Study the drawing (mm; zero at the part's minimum x, y, z) and answer. A direction names the side the tool comes from. Coordinates: 2 decimals unless noted, no trailing zeros. Order: outer loops, then holes, each group sorted by start corner. A loop starts at its lowest first (then second) coordinate and runs counter-clockwise, first axis right, second up. Notation, with made-up numbers: M -12.5,-35 L 22.5,-35 A27 cw 22.5,-8 Z; hole C 88,20 d9. An arc over 180 degrees is marked long. Use a Markdown table: item, result. Add a question column.
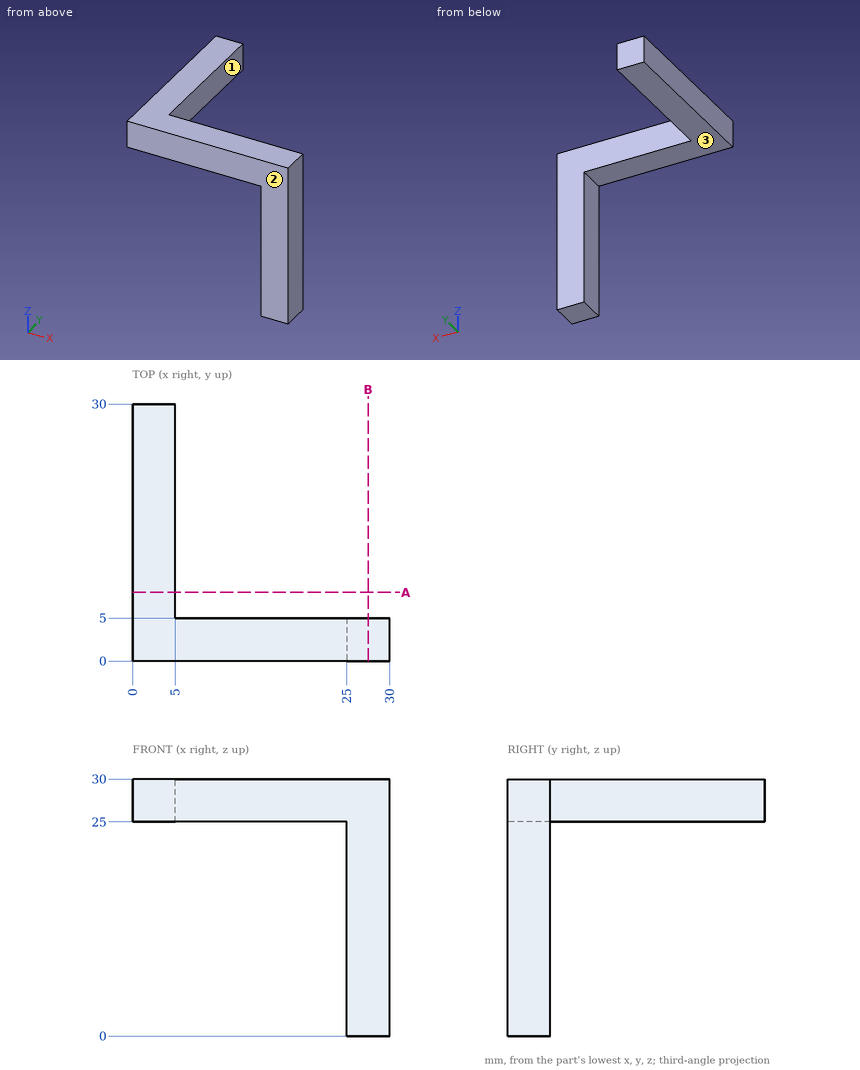
(1) A cutting plane is placed at A-A on y = 8. Write down the section's boundary in (x, z).
(2) Given P1, Ø2, axis at x = 20, y = 6.5, coming from the -Z side; P2, Ø5.5, axis at y = 2.5, z = 6.5, coming from the -X side; P3, Ø3, axis at x = 25.5, z = 14, coming from the +Y side; P4, Ø5.5, axis at y = 15.5, z = 28, coming from the +X side, each flat-ended and moving along its own axis, determine where each tip first touches the part or whether it passes through.
(3) Which of the six approach directions +Z, -Z, +X, -X, +Y, -Y give full straight-line access (tool end or side, diameter ignored) to the marked faces 1, 2 and 3?
(4) A cutting plane is placed at B-B on x = 27.5. Write down the section's boundary in (y, z).
(5) Straight lines are drawn through the part: line 1 (Y direction, x = 20.25, z = 25.5); line 2 (Z direction, x = 1.75, y = 9.75). For each, find the intervals that lie inside material, in ascending order.
From the geometry:
| question | item | result |
|---|---|---|
| 1 | outline | M 0,25 L 5,25 L 5,30 L 0,30 Z |
| 2 | P1 | passes through |
| 2 | P2 | stops at x = 25 |
| 2 | P3 | stops at y = 5 |
| 2 | P4 | stops at x = 5 |
| 3 | face 1 | +Z, -Z, +X, +Y |
| 3 | face 2 | +Z, -Z, +X, -X, -Y |
| 3 | face 3 | -Z, -X, +Y, -Y |
| 4 | outline | M 0,0 L 5,0 L 5,30 L 0,30 Z |
| 5 | line 1 | y = 0 to 5 |
| 5 | line 2 | z = 25 to 30 |
